from build123d import *

# Parameters (mm, degrees)
ESQUISSE1_W                                 = 103
ESQUISSE1_H                                 = 53
BOSS_EXTRU_1_DEPTH                          = 1.5
FRAISAGE_POUR_VIS_T_TE_FRAIS_E_M31_AT_COUNT = 2
FRAISAGE_POUR_VIS_T_TE_FRAIS_E_M31_AT_PITCH = 95.02
FRAISAGE_POUR_VIS_T_TE_FRAIS_E_M31_2_COUNT  = 2
FRAISAGE_POUR_VIS_T_TE_FRAIS_E_M31_2_PITCH  = 105.137055314
FRAISAGE_POUR_VIS_T_TE_FRAIS_E_M31_3_COUNT  = 2
FRAISAGE_POUR_VIS_T_TE_FRAIS_E_M31_3_PITCH  = 45
CONG_1_R                                    = 3.99
ESQUISSE4_R                                 = 2.9
ENL_V_MAT_EXTRU_1_DEPTH                     = 2.5


with BuildPart() as part:
    # Esquisse1 → Boss.-Extru.1 (new body)
    with BuildSketch(Plane(origin=(0, 0, -0.75), x_dir=(-1, 0, 0), z_dir=(0, 0, -1))):
        Rectangle(ESQUISSE1_W, ESQUISSE1_H)
    extrude(amount=-BOSS_EXTRU_1_DEPTH)

    # Esquisse2 → Fraisage pour vis à tête fraisée M31 (revolve, cut)
    with BuildSketch(Plane(origin=(-47.51, 22.5, 0.75), x_dir=(0, -1, 0), z_dir=(1, 0, 0))):
        Polygon((0, 0), (0, 1.5), (1.75, 1.5), (1.75, 1.125), (2.875, 0), align=None)
    fraisage_pour_vis_t_te_frais_e_m31 = revolve(axis=Axis((-47.51, 22.5, 7.1), (0, 0, -1)), mode=Mode.SUBTRACT)

    # Fraisage pour vis à tête fraisée M31 at: Fraisage pour vis à tête fraisée M31 ×2
    with Locations(*[(i * FRAISAGE_POUR_VIS_T_TE_FRAIS_E_M31_AT_PITCH, 0, 0) for i in range(1, FRAISAGE_POUR_VIS_T_TE_FRAIS_E_M31_AT_COUNT)]):
        add(fraisage_pour_vis_t_te_frais_e_m31, mode=Mode.SUBTRACT)

    # Fraisage pour vis _ t_te frais_e M31 2: Fraisage pour vis à tête fraisée M31 ×2
    with Locations(*[Vector(0.903772697, -0.428012748, 0) * (i * FRAISAGE_POUR_VIS_T_TE_FRAIS_E_M31_2_PITCH) for i in range(1, FRAISAGE_POUR_VIS_T_TE_FRAIS_E_M31_2_COUNT)]):
        add(fraisage_pour_vis_t_te_frais_e_m31, mode=Mode.SUBTRACT)

    # Fraisage pour vis _ t_te frais_e M31 3: Fraisage pour vis à tête fraisée M31 ×2
    with Locations(*[(0, -i * FRAISAGE_POUR_VIS_T_TE_FRAIS_E_M31_3_PITCH, 0) for i in range(1, FRAISAGE_POUR_VIS_T_TE_FRAIS_E_M31_3_COUNT)]):
        add(fraisage_pour_vis_t_te_frais_e_m31, mode=Mode.SUBTRACT)

    # Congé1
    cong_1_edges = [part.edges().sort_by_distance(p)[0] for p in [
        (51.5, 26.5, 0),
        (-51.5, 26.5, 0),
        (-51.5, -26.5, 0),
        (51.5, -26.5, 0),
    ]]
    fillet(cong_1_edges, radius=CONG_1_R)

    # Esquisse4 → Enlèv. mat.-Extru.1 (cut, through all)
    with BuildSketch(Plane.XY.offset(0.75)):
        with Locations((26.5, 12)):
            Circle(ESQUISSE4_R)
        with Locations((6.5, 12)):
            Circle(ESQUISSE4_R)
    extrude(amount=-ENL_V_MAT_EXTRU_1_DEPTH, mode=Mode.SUBTRACT)


solid = part.part
Can you work these out from the model? Positions are in its coordinate system, mm. Round coordinates to 2 decimals unless told otherwise and drop trailing zeros. Loops run counter-clockwise (first coordinate to the right, second up) from the corner with the lowest first, then second, coordinate; pieces in that order, holes last. Notation, with made-up numbers: (45, -4) - (80, -4) arc R28 ccw to (80, 21) - close; hole circle Ø5 at (13, 49.25). An arc over 180 degrees is marked (long way). Write item = value, one per line. Start each with the question number.
(1) If we section it at A-A (y = 12): Please give me the cut outline in (x, z).
(2) If we section it at C-C (z = 0.4): Please give me the cut outline in (x, y) (3 decimals), and give its area (3 significant figures).
(3) If we section it at B-B (x = 6.5): Please give me the cut outline in (y, z), and give its area (3 significant figures).
(4) If I drill on probe 1 along Y at (x, z) = (-47.51, -0.6); probe 2 along X at (y, z) = (-22.5, -0.45); probe 3 along Y at (x, z) = (6.5, -0.3), over which ranges is the centre line in solid material (lowest first)? Write a range as [from, to].
(5) If we mould it in two halves opening along X, with no side actions, what happens to faces 1 (the face through (1, 0, 0.75)), 2 (the face through (-50.3, -25.36, 0.01)), 3 (the face through (48.57, -21.11, -0.56))? For each: released by +X, released by -X, zero draft, split by the parting line, or undercut.
(6) For P1, Ø2, axis at x = -47.51, y = 22.5, coming from the -Z side; P2, Ø4.5, axis at x = -47.51, y = -22.5, coming from the +Z side (3 decimals), each with a flat end and sliding along its axis, tell me the tip position at first contact or that it passes through.
Ans:
q1.outline = (-51.5, -0.75) - (3.6, -0.75) - (3.6, 0.75) - (-51.5, 0.75) - close; (9.4, -0.75) - (23.6, -0.75) - (23.6, 0.75) - (9.4, 0.75) - close; (29.4, -0.75) - (51.5, -0.75) - (51.5, 0.75) - (29.4, 0.75) - close
q2.outline = (-51.5, -22.51) arc R3.99 ccw to (-47.51, -26.5) - (47.51, -26.5) arc R3.99 ccw to (51.5, -22.51) - (51.5, 22.51) arc R3.99 ccw to (47.51, 26.5) - (-47.51, 26.5) arc R3.99 ccw to (-51.5, 22.51) - close; hole circle Ø5.05 at (-47.51, -22.5); hole circle Ø5.05 at (-47.51, 22.5); hole circle Ø5.8 at (6.5, 12); hole circle Ø5.8 at (26.5, 12); hole circle Ø5.05 at (47.51, -22.5); hole circle Ø5.05 at (47.51, 22.5)
q2.area = 5,310 mm²
q3.outline = (-26.5, -0.75) - (9.1, -0.75) - (9.1, 0.75) - (-26.5, 0.75) - close; (14.9, -0.75) - (26.5, -0.75) - (26.5, 0.75) - (14.9, 0.75) - close
q3.area = 70.8 mm²
q4.probe_1 = [-26.5, -24.25], [-20.75, 20.75], [24.25, 26.5]
q4.probe_2 = [-51.5, -49.26], [-45.76, 45.76], [49.26, 51.5]
q4.probe_3 = [-26.5, 9.1], [14.9, 26.5]
q5.face_1 = zero draft
q5.face_2 = released by -X
q5.face_3 = undercut
q6.P1 = through
q6.P2 = 0.125
